The model under review builds one solid part; all positions refer to its coordinate system, in mm. A direction names the side the tool comes from. Coordinates: 2 decimals unless noted, no trailing zeros. Loops run counter-clockwise (first coordinate to the right, second up) from the corner with the lowest first, then second, coordinate; pieces in that order, holes last. Notation, with made-up numbers: M -4.5,-33.5 L -0.5,-33.5 A9 ccw -0.5,-21.5 Z; hole C -25,71.5 d11. An arc over 180 degrees is marked long. Use one line per item in the form item = value.
```python
from build123d import *

# Parameters (mm, degrees)
SKETCH1_W           = 25.4
SKETCH1_H           = 50.8
SKETCH1_W_2         = 20.32
SKETCH1_H_2         = 45.72
BOSS_EXTRUDE1_DEPTH = 76.2
SKETCH2_R           = 0.5
CUT_EXTRUDE1_DEPTH  = 76.2


with BuildPart() as part:
    # Sketch1 → Boss-Extrude1 (new body)
    with BuildSketch(Plane(origin=(0, 0, 0), x_dir=(1, 0, 0), z_dir=(0, 1, 0))):
        with Locations((12.7, 25.4)):
            Rectangle(SKETCH1_W, SKETCH1_H)
        with Locations((12.7, 25.4)):
            Rectangle(SKETCH1_W_2, SKETCH1_H_2, mode=Mode.SUBTRACT)
    extrude(amount=BOSS_EXTRUDE1_DEPTH)

    # Sketch2 → Cut-Extrude1 (cut)
    with BuildSketch(Plane(origin=(0, 0, -50.8), x_dir=(-1, 0, 0), z_dir=(0, 0, -1))):
        with Locations((-12.7, 12.7)):
            Circle(SKETCH2_R)
        with Locations((-12.7, 25.4)):
            Circle(SKETCH2_R)
        with Locations((-12.7, 38.1)):
            Circle(SKETCH2_R)
        with Locations((-12.7, 50.8)):
            Circle(SKETCH2_R)
        with Locations((-12.7, 63.5)):
            Circle(SKETCH2_R)
    extrude(amount=-CUT_EXTRUDE1_DEPTH, mode=Mode.SUBTRACT)


solid = part.part
```
1. Add section B-B (y = 52.5). State the section outline as (x, z) points, then the cut area to 3 significant figures.
Response values:
outline = M 0,-50.8 L 25.4,-50.8 L 25.4,0 L 0,0 Z; hole M 2.54,-48.26 L 22.86,-48.26 L 22.86,-2.54 L 2.54,-2.54 Z
area = 361 mm^2
2. Add section C-C (x = 5.5). State the section outline as (y, z) points, then the cut area to 3 significant figures.
Response values:
outline = M 0,-50.8 L 76.2,-50.8 L 76.2,-48.26 L 0,-48.26 Z; M 0,-2.54 L 76.2,-2.54 L 76.2,0 L 0,0 Z
area = 387 mm^2
3. Insertion check: P1, Ø5, axis at x = 18, z = -20, coming from the -Y side (3 decimals). The pin has a flat end and moves straight along its axis. Give the tip position at first contact, or say it passes through.
Response values:
P1 = through
4. Machinability: for faces 5 (the face through (2, 76.2, -27)), 6 (the face through (22.86, 38, -25)), which of the approach directions +Z, -Z, +X, -X, +Y, -Y give a long, thin tool a straight path to every point of the face, cutting with its end or side? Answer none if there is none.
Response values:
face_5 = +Z, -Z, +X, -X, +Y
face_6 = +Y, -Y
5. Add section A-A (z = -21). State the section outline as (x, y) points, then the cut area to 3 significant figures.
Response values:
outline = M 0,0 L 2.54,0 L 2.54,76.2 L 0,76.2 Z; M 22.86,0 L 25.4,0 L 25.4,76.2 L 22.86,76.2 Z
area = 387 mm^2
6. The part is to be moulded in two halves that separate along Z. For faces 1 (the face through (15, 38, -50.8)), 2 (the face through (2, 0, -27)), 3 (the face through (2.54, 38, -25)), 4 (the face through (10, 38, -48.26)), say which applies: pulls with the +Z half, pulls with the -Z half, needs draft (parallel to the pull), parting line crosses it, or undercut.
Response values:
face_1 = pulls with the -Z half
face_2 = needs draft
face_3 = undercut
face_4 = undercut
7. Wall thickness on line 1 along Y through (x, z) = (12.7, -1); line 2 along Z through (x, y) = (5, 43); line 3 along X through (y, z) = (52, -39.5): over which ranges is each line inside the solid? List them lowest first. Write a range as from..to.
Response values:
line_1 = 0..12.2, 13.2..24.9, 25.9..37.6, 38.6..50.3, 51.3..63, 64..76.2
line_2 = -50.8..-48.26, -2.54..0
line_3 = 0..2.54, 22.86..25.4
